```python
from build123d import *

# Parameters (mm, degrees)
BOSS_EXTRUDE1_DEPTH = 18
SKETCH2_R           = 3
CUT_EXTRUDE1_DEPTH  = 61


with BuildPart() as part:
    # Sketch1 → Boss-Extrude1 (new body)
    with BuildSketch(Plane(origin=(0, 0, 0), x_dir=(1, 0, 0), z_dir=(0, 1, 0))):
        with BuildLine():
            Line((-35, 30), (35, 30))
            Line((35, 30), (35, -30))
            Line((35, -30), (-35, -30))
            Line((-35, -30), (-35, -3))
            Line((-35, -3), (-19.773719933, -3))
            ThreePointArc((-19.773719933, -3), (20, 0), (-19.773719933, 3))
            Line((-19.773719933, 3), (-35, 3))
            Line((-35, 3), (-35, 30))
        make_face()
    extrude(amount=BOSS_EXTRUDE1_DEPTH)

    # Sketch2 → Cut-Extrude1 (cut, through all)
    with BuildSketch(Plane.XY.offset(30)):
        with Locations((27.5, 9)):
            Circle(SKETCH2_R)
        with Locations((-27.5, 9)):
            Circle(SKETCH2_R)
    extrude(amount=-CUT_EXTRUDE1_DEPTH, mode=Mode.SUBTRACT)


solid = part.part
```
The model under review builds one solid part; all positions refer to its coordinate system, in mm. A direction names the side the tool comes from. Round coordinates to 2 decimals unless told otherwise and drop trailing zeros. Order: outer loops, then holes, each group sorted by start corner. A loop starts at its lowest first (then second) coordinate and runs counter-clockwise, first axis right, second up.
(1) For P1, Ø6, axis at x = 17.5, z = 12.5, coming from the -Y side, flat-tipped, find the tip position at first contact; note if it passes through.
Working result:
P1: stops at y = 0
(2) Take a section at D-D, the plane x = 27.5. State the section outline as (y, z) points.
Working result:
outline: (0, -30) - (6, -30) - (6, 30) - (0, 30) - close; (12, -30) - (18, -30) - (18, 30) - (12, 30) - close
(3) Take a section at C-C, the plane x = -27.5. State the section outline as (y, z) points, plus the area to 3 significant figures.
Working result:
outline: (0, -30) - (6, -30) - (6, -3) - (0, -3) - close; (0, 3) - (6, 3) - (6, 30) - (0, 30) - close; (12, -30) - (18, -30) - (18, -3) - (12, -3) - close; (12, 3) - (18, 3) - (18, 30) - (12, 30) - close
area: 648 mm2
(4) Take a section at A-A, the plane y = 9. State the section outline as (x, z) points, plus the area to 3 significant figures.
Working result:
outline: (-35, -30) - (-30.5, -30) - (-30.5, -3) - (-35, -3) - close; (-35, 3) - (-30.5, 3) - (-30.5, 30) - (-35, 30) - close; (-24.5, -30) - (24.5, -30) - (24.5, 30) - (-24.5, 30) - (-24.5, 3) - (-19.77, 3) arc R20 cw (long way) to (-19.77, -3) - (-24.5, -3) - close; (30.5, -30) - (35, -30) - (35, 30) - (30.5, 30) - close
area: 2,170 mm2
(5) Wall thickness on L1, parallel to X at y = 8.75, z = 23.5; L2, parallel to X at y = 8.75, z = 0; L3, parallel to Z at x = 0, y = 4: over which ranges is each line inside the solid? List them lowest first.
Working result:
L1: x = -35 to -30.49, -24.51 to 24.51, 30.49 to 35
L2: x = 20 to 24.51, 30.49 to 35
L3: z = -30 to -20, 20 to 30
(6) Take a section at B-B, the plane z = -12.5. State the section outline as (x, y) points, plus the area to 3 significant figures.
Working result:
outline: (-35, 0) - (-15.61, 0) - (-15.61, 18) - (-35, 18) - close; (15.61, 0) - (35, 0) - (35, 18) - (15.61, 18) - close; hole circle Ø6 at (-27.5, 9); hole circle Ø6 at (27.5, 9)
area: 641 mm2
(7) Mouldability with a two-part tool opening along X and no side actions: class faces 3 (the face through (35, 9, 0)), 4 (the face through (-24, 9, 3)), 5 (the face through (-30.5, 9.1, 16.7)) as released by +X, released by -X, zero draft, split by the parting line, or undercut.
Working result:
face 3: released by +X
face 4: zero draft
face 5: undercut
(8) Tool access review of faces 1 (the face through (-31, 9, -3)), 2 (the face through (-35, 9, -16)): name each direction out of +Z, -Z, +X, -X, +Y, -Y from which nothing blocks a thin tool from reaching the whole face with its end or side.
Working result:
face 1: -X, +Y, -Y
face 2: +Z, -Z, -X, +Y, -Y
